Geometry: see drawing. Coordinates: mm, zero at the bounding-box minimum. A direction names the side the tool comes from. Coordinates: 2 decimals unless noted, no trailing zeros. Order: outer loops, then holes, each group sorted by start corner. A loop starts at its lowest first (then second) coordinate and runs counter-clockwise, first axis right, second up. Notation, with made-up numbers: (1, 61.25) -> (34, 61.25) arc R21 cw to (34, 100.25) -> close; hole circle Ø4 at (20.25, -17.5). An arc over 180 degrees is marked (long way). Use one line per item in the form item = value.
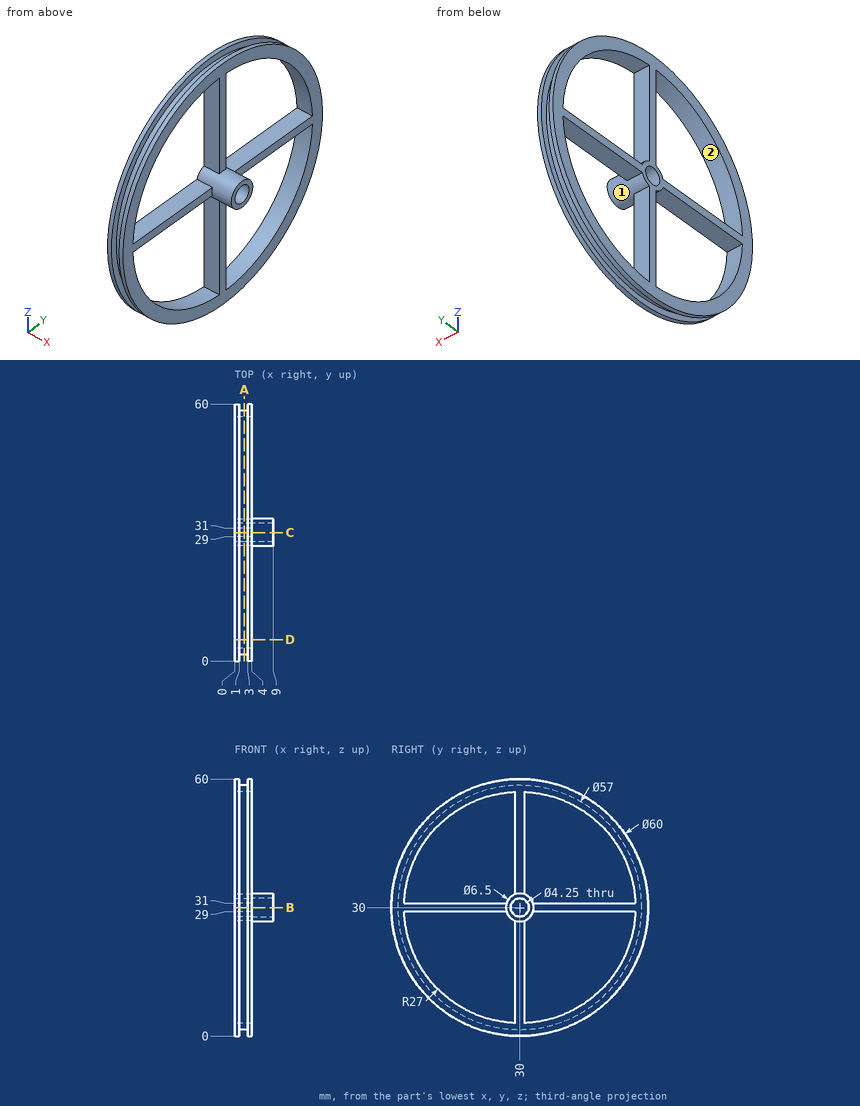
1) Section A-A, the plane x = 2.25. Output: boundary loops of the cut face in (y, z) (3 decimals), and give its area (3 significant figures).
Results found:
outline = circle Ø57 at (30, 30); hole (3.019, 29) arc R27 ccw to (29, 3.019) -> (29, 26.908) arc R3.25 cw to (26.908, 29) -> close; hole (3.019, 31) -> (26.908, 31) arc R3.25 cw to (29, 33.092) -> (29, 56.981) arc R27 ccw to start; hole circle Ø4.25 at (30, 30); hole (31, 3.019) arc R27 ccw to (56.981, 29) -> (33.092, 29) arc R3.25 cw to (31, 26.908) -> close; hole (31, 33.092) arc R3.25 cw to (33.092, 31) -> (56.981, 31) arc R27 ccw to (31, 56.981) -> close
area = 471 mm2
2) Section D-D, the plane y = 5. Output: boundary loops of the cut face in (x, z).
Results found:
outline = (0, 13.42) -> (1, 13.42) -> (1, 16.32) -> (3, 16.32) -> (3, 13.42) -> (4, 13.42) -> (4, 19.8) -> (0, 19.8) -> close; (0, 29) -> (4, 29) -> (4, 31) -> (0, 31) -> close; (0, 40.2) -> (4, 40.2) -> (4, 46.58) -> (3, 46.58) -> (3, 43.68) -> (1, 43.68) -> (1, 46.58) -> (0, 46.58) -> close
3) Section B-B, the plane z = 30. Output: boundary loops of the cut face in (x, y) (3 decimals), and give its area (3 significant figures).
Results found:
outline = (0, 0) -> (1, 0) -> (1, 1.5) -> (3, 1.5) -> (3, 0) -> (4, 0) -> (4, 26.75) -> (9, 26.75) -> (9, 27.875) -> (0, 27.875) -> close; (0, 32.125) -> (9, 32.125) -> (9, 33.25) -> (4, 33.25) -> (4, 60) -> (3, 60) -> (3, 58.5) -> (1, 58.5) -> (1, 60) -> (0, 60) -> close
area = 228 mm2
4) Material intervals for probe 1 along Z at (x, y) = (7, 30) (3 decimals); probe 2 along Y at (x, z) = (2.75, 22); probe 3 along Y at (x, z) = (2.25, 43), sorted ascending. Write a range as from..to.
Results found:
probe_1 = 26.75..27.875, 32.125..33.25
probe_2 = 2.65..4.21, 29..31, 55.79..57.35
probe_3 = 4.64..6.34, 29..31, 53.66..55.36
5) Access query for the marked faces 1 and 2. Directions: +Z, -Z, +X, -X, +Y, -Y. A direction counts if a zero-diameter tool reaches every point of the face in a straight line with its end or side. Return the directions, or none.
Results found:
face_1 = +X
face_2 = +X, -X
6) Contact query for flat-ended pins moving along their axis: P1, Ø3, axis at x = 1.5, z = 17, coming from the +Y side; P2, Ø4.5, axis at x = 2, z = 40, coming from the +Y side; P3, Ø4.5, axis at x = 1.5, y = 46, coming from the +Z side; P4, Ø7, axis at y = 30, z = 30, coming from the +X side. Output: stop coordinate, or through.
Results found:
P1 = 57.67
P2 = 58.92
P3 = 56.63
P4 = 9
